The model under review builds one solid part; all positions refer to its coordinate system, in mm. A direction names the side the tool comes from. Coordinates: 2 decimals unless noted, no trailing zeros. Loops run counter-clockwise (first coordinate to the right, second up) from the corner with the lowest first, then second, coordinate; pieces in that order, holes last. Notation, with made-up numbers: M -16,50.5 L 27,50.5 A21 ccw 27,73.5 Z; hole C -22,0.25 d4. An arc over 180 degrees is marked long. Return JSON: item names as keys, results as strings.
```python
from build123d import *

# Parameters (mm, degrees)
SKETCH_1_R          = 5
EXTRUDE_1_DEPTH     = 15
FILLET_1_R          = 3
SKETCH_2_R          = 2.5
CUT_EXTRUDE_1_DEPTH = 180.107509614
SKETCH_4_R          = 9.5
CUT_EXTRUDE_3_DEPTH = 20


with BuildPart() as part:
    # 草图1 → 凸台-拉伸1 (new body)
    with BuildSketch(Plane(origin=(0, 0, 0), x_dir=(1, 0, 0), z_dir=(0, 1, 0))):
        with BuildLine():
            Line((-17.971076762, -1.02), (-26.457418567, 148.498333333))
            ThreePointArc((-26.457418567, 148.498333333), (0, 176.5), (26.457418567, 148.498333333))
            Line((26.457418567, 148.498333333), (17.971076762, -1.02))
            ThreePointArc((17.971076762, -1.02), (0, -18), (-17.971076762, -1.02))
        make_face()
        with Locations(Location((0, 0, 0), (0, 0, 270))):
            Circle(SKETCH_1_R, mode=Mode.SUBTRACT)
        Polygon((-12.740980954, 12.714849757), (-18.554385191, 115.139490738), (10.712851955, 17.329399023), align=None, mode=Mode.SUBTRACT)
        Polygon((13.283215706, 22.268322657), (18.830257334, 120), (-12, 127), align=None, mode=Mode.SUBTRACT)
        with BuildLine():
            Line((0, 156.5), (4.663689527, 156.5))
            ThreePointArc((4.663689527, 156.5), (0, 142), (-4.663689527, 156.5))
            Line((-4.663689527, 156.5), (0, 156.5))
        make_face(mode=Mode.SUBTRACT)
    extrude(amount=EXTRUDE_1_DEPTH)

    # 圆角1
    fillet_1_edges = [part.edges().sort_by_distance(p)[0] for p in [
        (-12.740980954, 7.5, -12.714849757),
        (10.712851955, 7.5, -17.329399023),
        (-18.554385191, 7.5, -115.139490738),
        (18.830257334, 7.5, -120),
        (-12, 7.5, -127),
        (13.283215706, 7.5, -22.268322657),
    ]]
    fillet(fillet_1_edges, radius=FILLET_1_R)

    # 草图2 → 切除-拉伸1 (cut, through all)
    with BuildSketch(Plane(origin=(0, 15, 0), x_dir=(1, 0, 0), z_dir=(0, 1, 0))):
        with Locations(Location((0, 168.5, 0), (0, 0, 270))):
            Circle(SKETCH_2_R)
        with Locations(Location((13.081475452, 163.081475452, 0), (0, 0, 270))):
            Circle(SKETCH_2_R)
        with Locations(Location((18.5, 150, 0), (0, 0, 270))):
            Circle(SKETCH_2_R)
        with Locations(Location((13.081475452, 136.918524548, 0), (0, 0, 270))):
            Circle(SKETCH_2_R)
        with Locations(Location((0, 131.5, 0), (0, 0, 270))):
            Circle(SKETCH_2_R)
        with Locations(Location((-13.081475452, 136.918524548, 0), (0, 0, 270))):
            Circle(SKETCH_2_R)
        with Locations(Location((-18.5, 150, 0), (0, 0, 270))):
            Circle(SKETCH_2_R)
        with Locations(Location((-13.081475452, 163.081475452, 0), (0, 0, 270))):
            Circle(SKETCH_2_R)
    extrude(amount=-CUT_EXTRUDE_1_DEPTH, mode=Mode.SUBTRACT)

    # 草图4 → 切除-拉伸3 (cut)
    with BuildSketch(Plane.XZ):
        with Locations(Location((0, 0, 0), (0, 0, 270))):
            Circle(SKETCH_4_R)
    extrude(amount=-CUT_EXTRUDE_3_DEPTH, mode=Mode.SUBTRACT)


solid = part.part
```
1. The part is to be moulded in two halves that separate along X. For faces 3 (the face through (-14.692, 7.605, -92.776)), 4 (the face through (-22.155, 7.395, -72.693)), 5 (the face through (-11, 15, -102)), 6 (the face through (13.832, 7.605, -160.697)), say which applies: released by +X, released by -X, zero draft, split by the parting line, or undercut.
Check values:
{"face 3": "undercut", "face 4": "released by -X", "face 5": "zero draft", "face 6": "undercut"}
2. To check wall thickness, follow line 1 (X direction, y = 4.25, z = -150); line 2 (X direction, y = 10.5, z = -76); line 3 (X direction, y = 6.5, z = -148.5). State the ranges of each line that lie inside material, in increasing order.
Check values:
{"line 1": "-26.5 to -21, -16 to -8, 8 to 16, 21 to 26.5", "line 2": "-22.34 to -16.33, -6.84 to 0.31, 16.33 to 22.34", "line 3": "-26.46 to -20.5, -16.5 to -7.86, 7.86 to 16.5, 20.5 to 26.46"}
3. Machinability: for faces 1 (the face through (-14.993, 7.395, -52.393)), 2 (the face through (-11, 0, -102)), which of the approach directions +Z, -Z, +X, -X, +Y, -Y give a long, thin tool a straight path to every point of the face, cutting with its end or side? Answer none if there is none.
Check values:
{"face 1": "+Y, -Y", "face 2": "+Z, -Z, +X, -X, -Y"}
4. Insertion check: pin 1 Ø3 at (x, z) = (18.5, -150) entering from +Y; pin 2 Ø4 at (y, z) = (7, -87.5) entering from -X; pin 3 Ø4 at (x, y) = (-5, 9.5) entering from +Z; pin 4 Ø8 at (x, y) = (-12, 6) entering from +Z. Each pin has a flat end and moves straight along its axis. Give the tip position at first contact, or say it passes through.
Check values:
{"pin 1": "through", "pin 2": "x = -23.11", "pin 3": "z = 17.75", "pin 4": "z = 16.12"}
5. Add section A-A on z = -1.5. Give the boundary of the cut face in (x, y), plus the area to 3 significant figures.
Check values:
{"outline": "M -18.11,0 L -9.38,0 L -9.38,15 L -18.11,15 Z; M 9.38,0 L 18.11,0 L 18.11,15 L 9.38,15 Z", "area": "262 mm²"}
6. Add section B-B on x = 0. Give the boundary of the cut face in (y, z).
Check values:
{"outline": "M 0,-176.5 L 15,-176.5 L 15,-171 L 0,-171 Z; M 0,-166 L 15,-166 L 15,-156.5 L 0,-156.5 Z; M 0,-142 L 15,-142 L 15,-134 L 0,-134 Z; M 0,-129 L 15,-129 L 15,-124.28 L 0,-124.28 Z; M 0,-77.29 L 15,-77.29 L 15,-53.13 L 0,-53.13 Z; M 0,-15.22 L 15,-15.22 L 15,-9.5 L 0,-9.5 Z; M 0,9.5 L 15,9.5 L 15,18 L 0,18 Z"}
7. Add section D-D on z = -131.5. Give the boundary of the cut face in (x, y), plus the area to 3 significant figures.
Check values:
{"outline": "M -25.49,0 L -2.5,0 L -2.5,15 L -25.49,15 Z; M 2.5,0 L 25.49,0 L 25.49,15 L 2.5,15 Z", "area": "690 mm²"}
8. Add section C-C on y = 13. State how many separate pieces and enclosed holes the cut face has, plus the area to 3 significant figures.
Check values:
{"separate pieces": "1", "enclosed holes": "12", "area": "5,050 mm²"}
